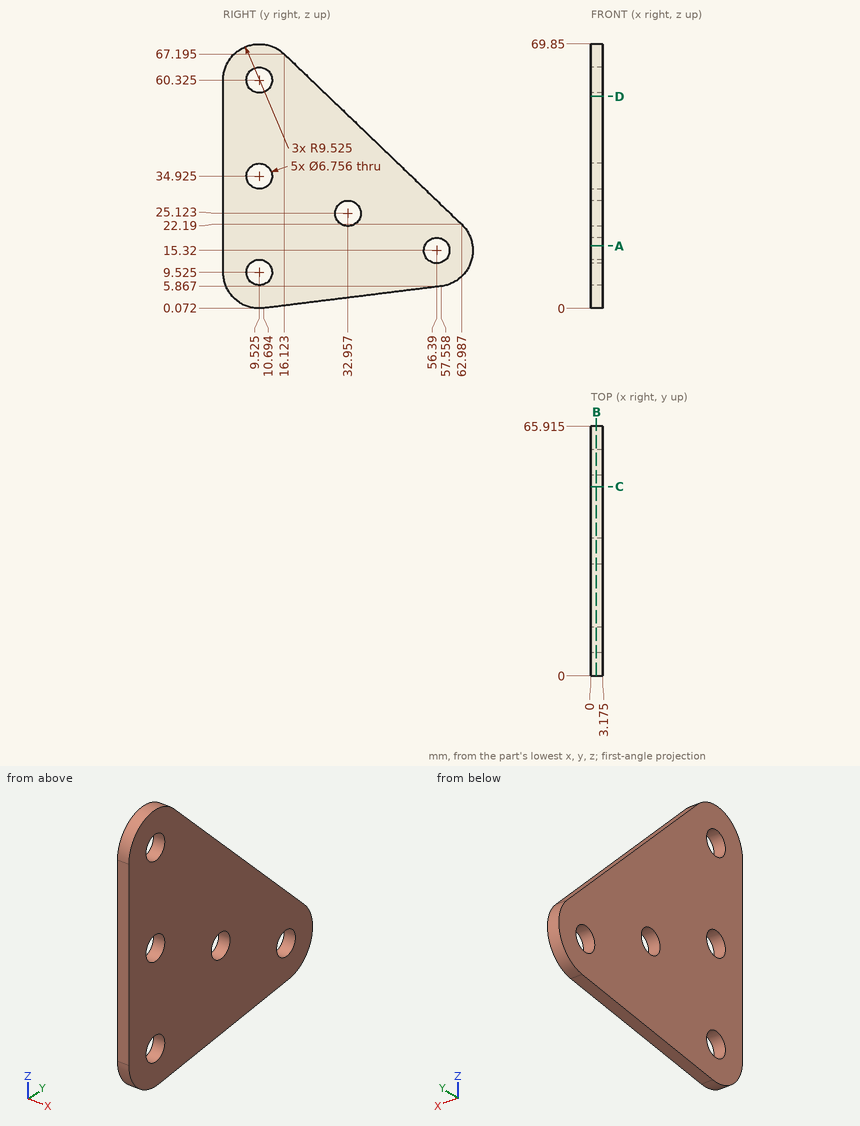
Verification items for this drawing (mm, ordinates from the low corner). Coordinates: 2 decimals unless noted, no trailing zeros. Loops run counter-clockwise (first coordinate to the right, second up) from the corner with the lowest first, then second, coordinate; pieces in that order, holes last.
Item 1: Sectioned sample at D-D, the plane z = 56. Record the boundary of the cut face in (x, y) (1 decimal).
Item 2: Sectioned sample at B-B, the plane x = 1.5. Count the separate pieces of the cut face and the enclosed holes in it, then the cut area to 3 significant figures.
Item 3: Sectioned sample at A-A, the plane z = 16.5. Record the boundary of the cut face in (x, y) (1 decimal), then the cut area to 3 significant figures.
Item 4: Thickness scan on line 1 (Z direction, x = 2.25, y = 10); line 2 (Z direction, x = 2.75, y = 8); line 3 (Y direction, x = 2.1, z = 35.5) (1 decimal). Record the ranges inside material, lowest first.
Item 5: Go/stop test with a flat-tipped pin: pin 1 Ø4 at (y, z) = (56.39, 15.32) entering from +X. Record where the tip stops, or that it passes through.
Item 6: Sectioned sample at C-C, the plane y = 50. Record the boundary of the cut face in (x, z) (1 decimal).
Check result:
1. outline: (0, 0) - (3.2, 0) - (3.2, 27.8) - (0, 27.8) - close
2. separate pieces: 1
2. enclosed holes: 5
2. area: 2,850 mm2
3. outline: (0, 0) - (3.2, 0) - (3.2, 53.2) - (0, 53.2) - close; (0, 59.6) - (3.2, 59.6) - (3.2, 65.8) - (0, 65.8) - close
3. area: 189 mm2
4. line 1: z = 0.01 to 6.18, 12.87 to 31.58, 38.27 to 56.98, 63.67 to 69.84
4. line 2: z = 0.12 to 6.51, 12.54 to 31.91, 37.94 to 57.31, 63.34 to 69.73
4. line 3: y = 0 to 6.2, 12.9 to 49.1
5. pin 1: passes through
6. outline: (0, 4.9) - (3.2, 4.9) - (3.2, 34.7) - (0, 34.7) - close
